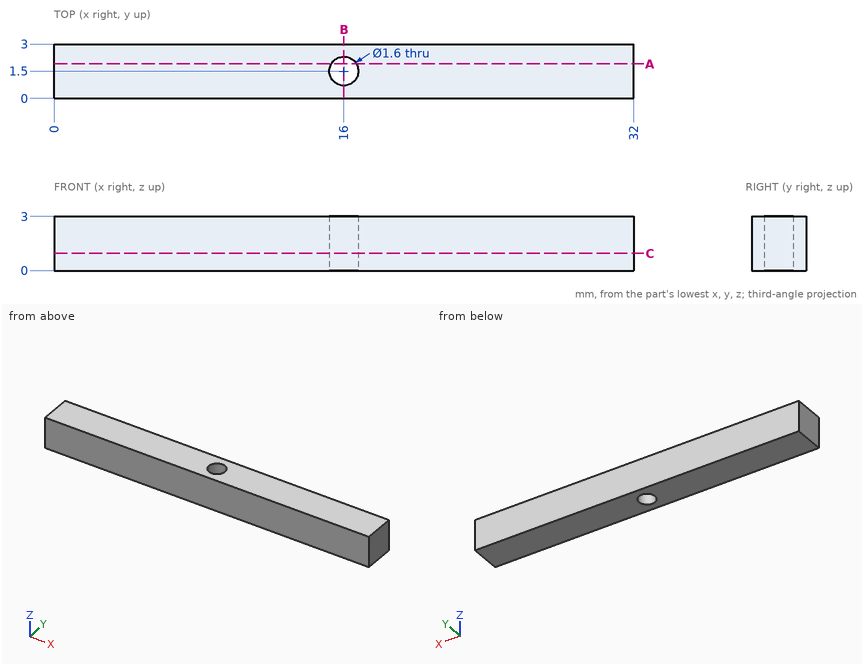
For this review, use the dimensioned drawing (mm, ordinates from the lowest corner) and the shaded views. Coordinates: 2 decimals unless noted, no trailing zeros. Loops run counter-clockwise (first coordinate to the right, second up) from the corner with the lowest first, then second, coordinate; pieces in that order, holes last. Notation, with made-up numbers: (70, 23.5) -> (125, 23.5) arc R22 cw to (125, 51.5) -> close; hole circle Ø3 at (15.25, 24). An arc over 180 degrees is marked (long way). Use a Markdown table: item, result. Add a question column.
Item 1: We need section A-A, the plane y = 1.9. Write out the cut boundary in (x, z).
Item 2: We need section C-C, the plane z = 0.95. Write out the cut boundary in (x, y), and give its area (3 significant figures).
Item 3: We need section B-B, the plane x = 16. Write out the cut boundary in (y, z).
Item 4: Clearance check with a flat-ended pin moving along its axis: P1, Ø1, axis at x = 3.5, y = 2, coming from the -Z side. State where the tip first meets the part, or that it passes through.
Item 5: Wall thickness on L1, parallel to Y at x = 16, z = 2.15; L2, parallel to X at y = 1.35, z = 2.05; L3, parallel to X at y = 0.8, z = 0.4: over which ranges is each line inside the solid? List them lowest first. Write a range as from..to.
Numbers:
| question | item | result |
|---|---|---|
| 1 | outline | (0, 0) -> (15.31, 0) -> (15.31, 3) -> (0, 3) -> close; (16.69, 0) -> (32, 0) -> (32, 3) -> (16.69, 3) -> close |
| 2 | outline | (0, 0) -> (32, 0) -> (32, 3) -> (0, 3) -> close; hole circle Ø1.6 at (16, 1.5) |
| 2 | area | 94.0 mm^2 |
| 3 | outline | (0, 0) -> (0.7, 0) -> (0.7, 3) -> (0, 3) -> close; (2.3, 0) -> (3, 0) -> (3, 3) -> (2.3, 3) -> close |
| 4 | P1 | stops at z = 0 |
| 5 | L1 | y = 0..0.7, 2.3..3 |
| 5 | L2 | x = 0..15.21, 16.79..32 |
| 5 | L3 | x = 0..15.61, 16.39..32 |
